Autodesk Inventor part; units mm, degrees
ref_plane "terminal_to_body_XY" through (0, 16.9926, 0) normal (0, 1, 0) x (1, 0, 0)
ref_plane "terminal_to_body_YZ" through (0, 16.9926, 0) normal (1, 0, 0) x (0, 0, -1)
ref_plane "terminal_to_body_ZX" through (0, 16.9926, 0) normal (0, 0, -1) x (0, 1, 0)
sketch "Sketch_1" plane through (0, 0.508, 0) normal (0, 1, 0) x (1, 0, 0)
  circle A0 centre (0, 0) radius 7.619
extrude "Extrusion1" add sketch "Sketch_1" along normal blind 0.4877
sketch "Sketch_8" plane through (1.8542, 0, 0) normal (1, 0, 0) x (0, 0, -1)
  line L0 (-1.397, -6.5532) -> (-0.635, -7.3152)
  line L1 (-0.635, -7.3152) -> (0.635, -7.3152)
  line L2 (0.635, -7.3152) -> (1.397, -6.5532)
  line L3 (1.397, -6.5532) -> (1.397, 0.762)
  line L4 (1.397, 0.762) -> (-1.397, 0.762)
  line L5 (-1.397, 0.762) -> (-1.397, -6.5532)
  line L6 (-0.5969, -4.8768) -> (-0.5969, -5.6896)
  arc A0 (-0.5969, -5.6896) -> (0.5969, -5.6896) centre (0, -5.6896) ccw
  line L7 (0.5969, -5.6896) -> (0.5969, -4.8768)
  arc A1 (0.5969, -4.8768) -> (-0.5969, -4.8768) centre (0, -4.8768) ccw
extrude "Extrusion2" add sketch "Sketch_8" along normal mid plane 0.508
sketch "Sketch_7" plane through (-1.8542, 0, 0) normal (1, 0, 0) x (0, 0, -1)
  line L0 (-1.397, -6.5532) -> (-0.635, -7.3152)
  line L1 (-0.635, -7.3152) -> (0.635, -7.3152)
  line L2 (0.635, -7.3152) -> (1.397, -6.5532)
  line L3 (1.397, -6.5532) -> (1.397, 0.762)
  line L4 (1.397, 0.762) -> (-1.397, 0.762)
  line L5 (-1.397, 0.762) -> (-1.397, -6.5532)
  line L6 (-0.5969, -4.8768) -> (-0.5969, -5.6896)
  arc A0 (-0.5969, -5.6896) -> (0.5969, -5.6896) centre (0, -5.6896) ccw
  line L7 (0.5969, -5.6896) -> (0.5969, -4.8768)
  arc A1 (0.5969, -4.8768) -> (-0.5969, -4.8768) centre (0, -4.8768) ccw
extrude "Extrusion3" add sketch "Sketch_7" along normal mid plane 0.508
sketch "Sketch_9" plane through (-5.5499, 0, 0) normal (1, 0, 0) x (0, 0, -1)
  line L0 (-1.397, -6.5532) -> (-0.635, -7.3152)
  line L1 (-0.635, -7.3152) -> (0.635, -7.3152)
  line L2 (0.635, -7.3152) -> (1.397, -6.5532)
  line L3 (1.397, -6.5532) -> (1.397, 0.762)
  line L4 (1.397, 0.762) -> (-1.397, 0.762)
  line L5 (-1.397, 0.762) -> (-1.397, -6.5532)
  line L6 (-0.5969, -4.8768) -> (-0.5969, -5.6896)
  arc A0 (-0.5969, -5.6896) -> (0.5969, -5.6896) centre (0, -5.6896) ccw
  line L7 (0.5969, -5.6896) -> (0.5969, -4.8768)
  arc A1 (0.5969, -4.8768) -> (-0.5969, -4.8768) centre (0, -4.8768) ccw
extrude "Extrusion4" add sketch "Sketch_9" along normal mid plane 0.508
sketch "Sketch_2" plane through (0, 0, 4.8514) normal (0, 0, 1) x (1, 0, 0)
  line L0 (-4.3942, -6.5532) -> (-3.6322, -7.3152)
  line L1 (-3.6322, -7.3152) -> (-2.3622, -7.3152)
  line L2 (-2.3622, -7.3152) -> (-1.6002, -6.5532)
  line L3 (-1.6002, -6.5532) -> (-1.6002, 0.762)
  line L4 (-1.6002, 0.762) -> (-4.3942, 0.762)
  line L5 (-4.3942, 0.762) -> (-4.3942, -6.5532)
  line L6 (-3.5941, -4.8768) -> (-3.5941, -5.6896)
  arc A0 (-3.5941, -5.6896) -> (-2.4003, -5.6896) centre (-2.9972, -5.6896) ccw
  line L7 (-2.4003, -5.6896) -> (-2.4003, -4.8768)
  arc A1 (-2.4003, -4.8768) -> (-3.5941, -4.8768) centre (-2.9972, -4.8768) ccw
extrude "Extrusion5" add sketch "Sketch_2" along normal mid plane 0.508
sketch "Sketch_11" plane through (0, 0, -4.8514) normal (0, 0, 1) x (1, 0, 0)
  line L0 (-4.3942, -6.5532) -> (-3.6322, -7.3152)
  line L1 (-3.6322, -7.3152) -> (-2.3622, -7.3152)
  line L2 (-2.3622, -7.3152) -> (-1.6002, -6.5532)
  line L3 (-1.6002, -6.5532) -> (-1.6002, 0.762)
  line L4 (-1.6002, 0.762) -> (-4.3942, 0.762)
  line L5 (-4.3942, 0.762) -> (-4.3942, -6.5532)
  line L6 (-3.5941, -4.8768) -> (-3.5941, -5.6896)
  arc A0 (-3.5941, -5.6896) -> (-2.4003, -5.6896) centre (-2.9972, -5.6896) ccw
  line L7 (-2.4003, -5.6896) -> (-2.4003, -4.8768)
  arc A1 (-2.4003, -4.8768) -> (-3.5941, -4.8768) centre (-2.9972, -4.8768) ccw
extrude "Extrusion6" add sketch "Sketch_11" along normal mid plane 0.508
ref_plane "terminal_to_body_XY" through (0, 16.9926, 0) normal (0, 1, 0) x (1, 0, 0)
ref_plane "terminal_to_body_YZ" through (0, 16.9926, 0) normal (1, 0, 0) x (0, 0, -1)
ref_plane "terminal_to_body_ZX" through (0, 16.9926, 0) normal (0, 0, -1) x (0, 1, 0)
properties part number "YB16SKW01-05-BBterminal"
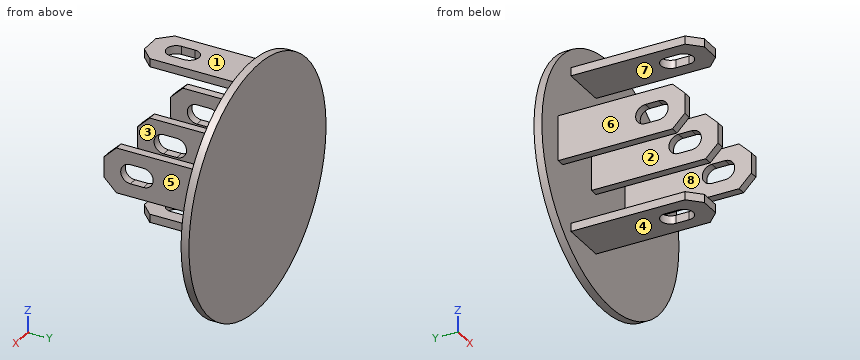
Check sheet for the modelled part. Datum: model origin and axes. Units: mm. Face numbers are marked on the shaded views. A direction names the side the tool comes from. Coordinates: 2 decimals unless noted, no trailing zeros. Write each loop counter-clockwise with the first axis right and the second up, starting at its lowest first coordinate (ties: lowest second). Pieces come first, ordered by that corner, then holes. Notation, with made-up numbers: M 61.5,5.5 L 95.5,5.5 A17 ccw 95.5,9.5 Z; hole C 14,-34.75 d3. An arc over 180 degrees is marked long. Answer as CSV lines item,"result".
Q1. Go/stop test with flat-tipped pins: pin 1 (3 mm diameter, centred on x = -3.5, y = -1.5, fed in from +Z); pin 2 (1.4 mm diameter, centred on y = -3.5, z = 0.5, fed in from +X); pin 3 (1 mm diameter, centred on y = -2, z = -4.5, fed in from +X). Record where each tip stops, or that it passes through.
Check result:
pin 1,"z = 5.11"
pin 2,"x = 2.11"
pin 3,"x = -1.6"
Q2. Cross-section at C-C (x = 0). Record the boundary of the cut face in (y, z), then the cut area to 3 significant figures.
Check result:
outline,"M 0.51,-7.62 L 1,-7.62 L 1,7.62 L 0.51,7.62 Z"
area,"7.43 mm^2"
Q3. Cross-section at A-A (y = -3). Record the boundary of the cut face in (x, z).
Check result:
outline,"M -5.8,-1.4 L -5.3,-1.4 L -5.3,1.4 L -5.8,1.4 Z; M -4.39,-5.11 L -1.6,-5.11 L -1.6,-4.6 L -4.39,-4.6 Z; M -4.39,4.6 L -1.6,4.6 L -1.6,5.11 L -4.39,5.11 Z; M -2.11,-1.4 L -1.6,-1.4 L -1.6,1.4 L -2.11,1.4 Z; M 1.6,-1.4 L 2.11,-1.4 L 2.11,1.4 L 1.6,1.4 Z"
Q4. Cross-section at D-D (y = -6). Count the separate pieces of the cut face and the enclosed holes in it, then the cut area to 3 significant figures.
Check result:
separate pieces,"10"
enclosed holes,"0"
area,"4.51 mm^2"
Q5. Mould release check, pull along X, two halves, no side actions. Record for the marked faces 6, 7 and 8: released by +X, released by -X, zero draft, split by the parting line, or undercut.
Check result:
face 6,"released by -X"
face 7,"zero draft"
face 8,"undercut"
Q6. Material ranges on probe 1 along X at (y, z) = (-5.5, -0.75); probe 2 along Z at (x, y) = (-5.5, -5.5); probe 3 along Z at (x, y) = (-3.75, -6.25), recorded low to high. Write a range as from..to.
Check result:
probe 1,"-5.8..-5.3, -2.11..-1.6, 1.6..2.11"
probe 2,"-1.4..-0.6, 0.6..1.4"
probe 3,"-5.11..-4.6, 4.6..5.11"
Q7. Cross-section at B-B (z = 0). Record the boundary of the cut face in (x, y), then the cut area to 3 significant figures.
Check result:
outline,"M -7.62,0.51 L -5.8,0.51 L -5.8,-4.28 L -5.3,-4.28 L -5.3,0.51 L -2.11,0.51 L -2.11,-4.28 L -1.6,-4.28 L -1.6,0.51 L 1.6,0.51 L 1.6,-4.28 L 2.11,-4.28 L 2.11,0.51 L 7.62,0.51 L 7.62,1 L -7.62,1 Z; M -5.8,-7.32 L -5.3,-7.32 L -5.3,-6.29 L -5.8,-6.29 Z; M -2.11,-7.32 L -1.6,-7.32 L -1.6,-6.29 L -2.11,-6.29 Z; M 1.6,-7.32 L 2.11,-7.32 L 2.11,-6.29 L 1.6,-6.29 Z"
area,"16.3 mm^2"
Q8. Set-up check for the marked faces 1, 2, 3, 4 and 5: record each of +Z, -Z, +X, -X, +Y, -Y from which the full face is reachable in a straight line by a thin tool's end or side.
Check result:
face 1,"+Z, +X, -X, -Y"
face 2,"-Y"
face 3,"+Z, -Z, -Y"
face 4,"-Z, +X, -X, -Y"
face 5,"+Z, -Z, +X, -Y"
